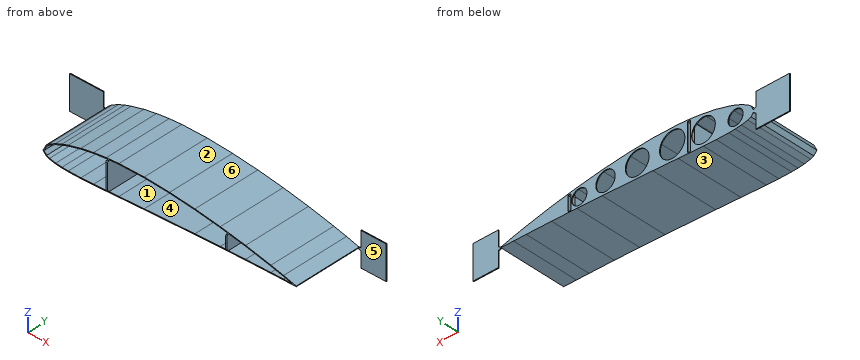
```python
from build123d import *

# Parameters (mm, degrees)
F1_DEPTH  = 40
F3_DEPTH  = 39.5
F4_R      = 4.5
F4_R_2    = 7
F4_R_3    = 7.5
F4_R_4    = 5.75
F5_DEPTH  = 0.501
F7_DEPTH  = 2
F8_W      = 1.75
F8_H      = 8.804983391
F8_W_2    = 2
F8_H_2    = 16.691370044
F9_DEPTH  = 1.25
F10_R     = 0.5
F11_W     = 0.75
F11_H     = 8.010983391
F11_W_2   = 1
F11_H_2   = 15.8301910942
F12_DEPTH = 1
F13_R     = 0.5
F15_DEPTH = 0.5
F17_DEPTH = 0.5


with BuildPart() as f1:
    # F0 (on Front) → F1 (new body)
    with BuildSketch(Plane.XZ):
        Polygon((150, -0.195), (150, 0.195), (142.5, 2.205), (135, 4.065), (120, 7.335), (105, 10.035), (90, 12.21), (75, 13.785), (60, 14.7), (45, 14.64), (37.5, 14.115), (30, 13.2), (22.5, 11.835), (15, 9.885), (11.25, 8.64), (7.5, 7.095), (3.75, 5.085), (1.875, 3.66), (0, 0), (1.875, -2.145), (3.75, -2.925), (7.5, -3.735), (11.25, -4.11), (15, -4.29), (22.5, -4.32), (30, -4.11), (37.5, -3.75), (45, -3.39), (60, -2.7), (75, -2.1), (90, -1.5), (105, -0.975), (120, -0.585), (135, -0.33), (142.5, -0.24), align=None)
    extrude(amount=F1_DEPTH)

    # F2 (on face) → F3 (cut)
    with BuildSketch(Plane.XZ.offset(40)):
        Polygon((22.494001199, -3.8199719571), (29.9810146479, -3.6103355805), (38.0995951893, -3.2206437145), (38.0995951893, 13.6557481124), (37.5477644894, 13.6171199634), (30.0751046996, 12.705455469), (22.6078220145, 11.3464100203), (15.1418358981, 9.4052536301), (11.4242210448, 8.1710054988), (7.7138856453, 6.6423473142), (4.0210598526, 4.6629926893), (2.2681271547, 3.3307638389), (0.5995951893, 0.0737894424), (2.1747084318, -1.728140107), (3.9000375829, -2.4458770339), (7.577907371, -3.2402969081), (11.2868867814, -3.6111948491), (15.0129924699, -3.7900479222), align=None)
        Polygon((89.9812632263, -1.0003495831), (104.9847572408, -0.4752272926), (109.0995951893, -0.3682415059), (109.0995951893, 8.7890373856), (104.9198136118, 9.5413980696), (89.9379946481, 11.7137618193), (74.958652077, 13.2865927893), (59.985763287, 14.1999390054), (45.0184773208, 14.1400698616), (39.0995951893, 13.7257481124), (39.0995951893, -3.1726437145), (44.9765259223, -2.8905510394), (59.9785199435, -2.2004593144), align=None)
        Polygon((109.8495951893, -0.3487415059), (119.9892525914, -0.0851104134), (134.992750784, 0.1699490558), (142.4955002021, 0.2599820488), (147.7092928365, 0.2912648047), (142.3750957537, 1.7208296229), (134.8865506068, 3.5779888193), (119.9024297861, 6.8445271582), (109.8495951893, 8.6540373856), align=None)
    extrude(amount=-F3_DEPTH, mode=Mode.SUBTRACT)

    # F4 (on face) → F5 (cut, through all)
    with BuildSketch(Plane.XZ.offset(0.5)):
        with Locations((11, 2)):
            Circle(F4_R)
        with Locations((30, 4.5)):
            Circle(F4_R_2)
        with Locations((48.5, 5.75)):
            Circle(F4_R_3)
        with Locations((69.25, 6)):
            Circle(F4_R_2)
        with Locations((88, 5.5)):
            Circle(F4_R_4)
        with Locations((103.5, 4.5)):
            Circle(F4_R)
    extrude(amount=-F5_DEPTH, mode=Mode.SUBTRACT)

    # F6 (on face) → F7 (join)
    with BuildSketch(Plane(origin=(0, 0, 0), x_dir=(-1, 0, 0), z_dir=(0, 1, 0))):
        Polygon((-110.8495951893, -0.8229105251), (-108.0995951893, -0.8944105251), (-108.0995951893, 9.4770728659), (-110.8495951893, 8.9820728659), align=None)
        Polygon((-37.0995951893, -3.7692194309), (-37.0995951893, 14.0661506131), (-37.5, 14.115), (-40.0995951893, 14.2969716633), (-40.0995951893, -3.6252194309), align=None)
    extrude(amount=-F7_DEPTH)

    # F8 (on face) → F9 (cut)
    with BuildSketch(Plane(origin=(0, 0, 0), x_dir=(-1, 0, 0), z_dir=(0, 1, 0))):
        with Locations((-109.4745951893, 4.0795811704)):
            Rectangle(F8_W, F8_H)
        with Locations((-38.5995951893, 5.2204655911)):
            Rectangle(F8_W_2, F8_H_2)
    extrude(amount=-F9_DEPTH, mode=Mode.SUBTRACT)

    # F10
    f10_edges = [f1.edges().sort_by_distance(p)[0] for p in [
        (37.599595, -1.25, 5.220466),
        (38.599595, -1.25, 13.566151),
        (39.599595, -1.25, 5.220466),
        (38.599595, -1.25, -3.125219),
        (108.599595, -1.25, 4.079581),
        (109.474595, -1.25, 8.482073),
        (110.349595, -1.25, 4.079581),
        (109.474595, -1.25, -0.322911),
    ]]
    fillet(f10_edges, radius=F10_R)

    # F11 (on face) → F12 (join)
    with BuildSketch(Plane.XZ.offset(40)):
        with Locations((109.4745951893, 4.1565811704)):
            Rectangle(F11_W, F11_H)
        with Locations((38.5995951893, 5.2418761162)):
            Rectangle(F11_W_2, F11_H_2)
    extrude(amount=F12_DEPTH)

    # F13
    f13_edges = [f1.edges().sort_by_distance(p)[0] for p in [
        (38.599595, -41, 13.156972),
        (38.599595, -41, -2.673219),
        (109.474595, -41, 0.151089),
        (109.474595, -41, 8.162073),
    ]]
    fillet(f13_edges, radius=F13_R)

    # F14 (on face) → F15 (join)
    with BuildSketch(Plane(origin=(0, 0, 0), x_dir=(-1, 0, 0), z_dir=(0, 1, 0))):
        Polygon((21, 10), (1, 10), (1, 1.8028106709), (-0.484496124, 0.9457364341), (0, 0), (-0.484496124, -0.5542635659), (1, -1.4113378027), (1, -10), (21, -10), align=None)
    extrude(amount=-F15_DEPTH)

    # F16 (on face) → F17 (join)
    with BuildSketch(Plane(origin=(0, 0, 0), x_dir=(-1, 0, 0), z_dir=(0, 1, 0))):
        Polygon((-151.5, 1.0610254038), (-151.5, 10), (-166.5, 10), (-166.5, -10), (-151.5, -10), (-151.5, -1.0610254038), (-150, -0.195), (-150, 0.195), align=None)
    extrude(amount=-F17_DEPTH)


solid = f1.part
```
Check sheet for the modelled part. Datum: model origin and axes. Units: mm. Face numbers are marked on the shaded views. A direction names the side the tool comes from. Round coordinates to 2 decimals unless told otherwise and drop trailing zeros. Order: outer loops, then holes, each group sorted by start corner. A loop starts at its lowest first (then second) coordinate and runs counter-clockwise, first axis right, second up. Notation, with made-up numbers: (-1.5, 75) -> (36.5, 75) arc R30 ccw to (36.5, 98) -> close; hole circle Ø11 at (10, -15). An arc over 180 degrees is marked (long way). Use CSV: the item, a comma, the result in double quotes.
(1) Draft check along Z on the marked faces 1, 2 and 3. Enter one of: pulls with the +Z half, pulls with the -Z half, needs draft (parallel to the pull), parting line crosses it, or undercut.
Worked out:
face 1,"undercut"
face 2,"pulls with the +Z half"
face 3,"pulls with the -Z half"
(2) Cross-section at C-C (y = -35.5). Count the separate pieces of the cut face and the enclosed holes in it, and give its area (3 significant figures).
Worked out:
separate pieces,"1"
enclosed holes,"3"
area,"176 mm²"
(3) Cross-section at A-A (z = -6.5). Record the boundary of the cut face in (x, y), and give its area (3 significant figures).
Worked out:
outline,"(-21, -0.5) -> (-1, -0.5) -> (-1, 0) -> (-21, 0) -> close; (151.5, -0.5) -> (166.5, -0.5) -> (166.5, 0) -> (151.5, 0) -> close"
area,"17.5 mm²"
(4) Material ranges on line 1 along Y through (x, z) = (63, 13.75); line 2 along Z through (x, y) = (15.5, -7) (3 decimals); line 3 along Z through (x, y) = (96, -19.5), recorded low to high. Write a range as from..to.
Worked out:
line 1,"-0.5..0"
line 2,"-4.292..-3.792, 9.498..10.015"
line 3,"-1.29..-0.79, 10.83..11.34"
(5) Tool access check on the marked faces 4, 5 and 6. Record the directions out of +Z, -Z, +X, -X, +Y, -Y that give a thin tool (end or side, any length) a straight path to the whole face; none if there is none.
Worked out:
face 4,"-Y"
face 5,"+Z, -Z, +X, -Y"
face 6,"+Z, +X, +Y, -Y"
(6) Cross-section at B-B (x = 48.5). Record the boundary of the cut face in (y, z), and give its area (3 significant figures).
Worked out:
outline,"(-40, -3.23) -> (0, -3.23) -> (0, -1.75) -> (-0.5, -1.75) -> (-0.5, -2.73) -> (-40, -2.73) -> close; (-40, 14.15) -> (-0.5, 14.15) -> (-0.5, 13.25) -> (0, 13.25) -> (0, 14.65) -> (-40, 14.65) -> close"
area,"41.0 mm²"
(7) Cross-section at D-D (x = 88). Record the boundary of the cut face in (y, z).
Worked out:
outline,"(-40, -1.58) -> (0, -1.58) -> (0, -0.25) -> (-0.5, -0.25) -> (-0.5, -1.08) -> (-40, -1.08) -> close; (-40, 11.92) -> (-0.5, 11.92) -> (-0.5, 11.25) -> (0, 11.25) -> (0, 12.42) -> (-40, 12.42) -> close"
(8) Depth check by flat-ended pin: pin 1 (0.5 mm diameter, centred on x = 108.5, z = 3, fed in from -Y); pin 2 (6 mm diameter, centred on y = -31.5, z = 9.5, fed in from -X); pin 3 (5 mm diameter, centred on x = 26, z = 0.5, fed in from -Y); pin 4 (3 mm diameter, centred on x = 15, z = 12, fed in from +Y). Enter the tip coordinate at first touch or a pass-through.
Worked out:
pin 1,"y = -2"
pin 2,"x = 6.39"
pin 3,"y = -0.5"
pin 4,"through"
